Source: three-view drawing plus pictorial views. Frame: mm from the lowest corner of the part. A direction names the side the tool comes from. Round coordinates to 2 decimals unless told otherwise and drop trailing zeros. Use one line per item in the form item = value. Start each with the question number.
Q1. Draft query along X for the marked faces 3, 4, 5 and 6. Return one class per face: released by +X, released by -X, zero draft, split by the parting line, or undercut.
Q2. Set-up query: the marked faces 1 and 2. Return all of +Z, -Z, +X, -X, +Y, -Y with unobstructed straight access to the full face (end or side cutting, diameter ignored); none if empty.
Q3. Cut plane C-C, the plane x = 7.75. Give the number of separate pieces and of enclosed holes in the cut face.
Q4. Ray query, line 1 (Z direction, x = 9.5, y = 2.75); line 2 (Y direction, x = 9, z = 17.5) (1 decimal). Return the intervals inside material, ascending. Write a range as [from, to].
Q5. Pin query (flat end, axial travel): pin 1 Ø7.5 at (x, z) = (9.52, 11.11) entering from +Y (1 decimal); pin 2 Ø5 at (x, y) = (7.5, 9.5) entering from +Z (1 decimal); pin 3 Ø5.5 at (x, y) = (9.52, 17.46) entering from +Z. Return the tip coordinate at first contact, or that it passes through.
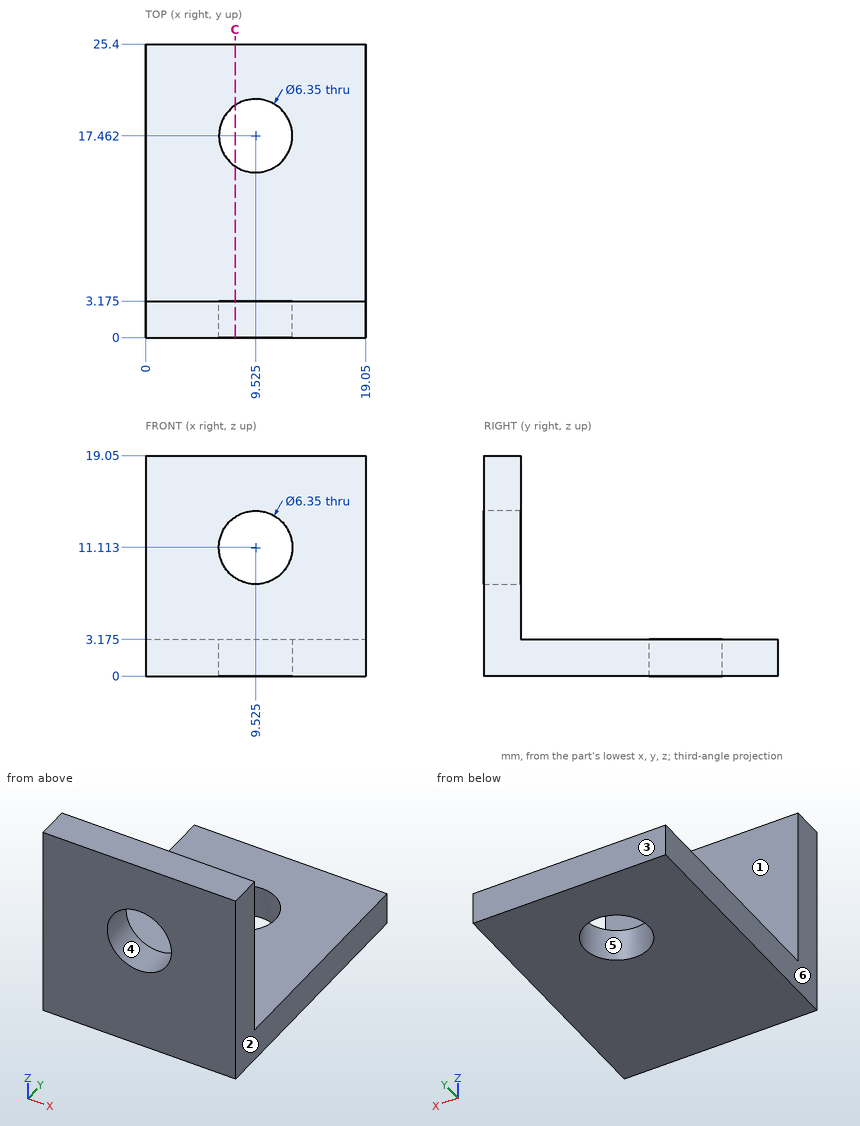
Completed:
q1.face_3 = zero draft
q1.face_4 = undercut
q1.face_5 = undercut
q1.face_6 = released by -X
q2.face_1 = +Z, +X, -X, +Y
q2.face_2 = +Z, -Z, +X, +Y, -Y
q3.separate_pieces = 3
q3.enclosed_holes = 0
q4.line_1 = [0, 7.94], [14.29, 19.05]
q4.line_2 = [0, 3.2]
q5.pin_1 = 3.2
q5.pin_2 = 3.2
q5.pin_3 = through
